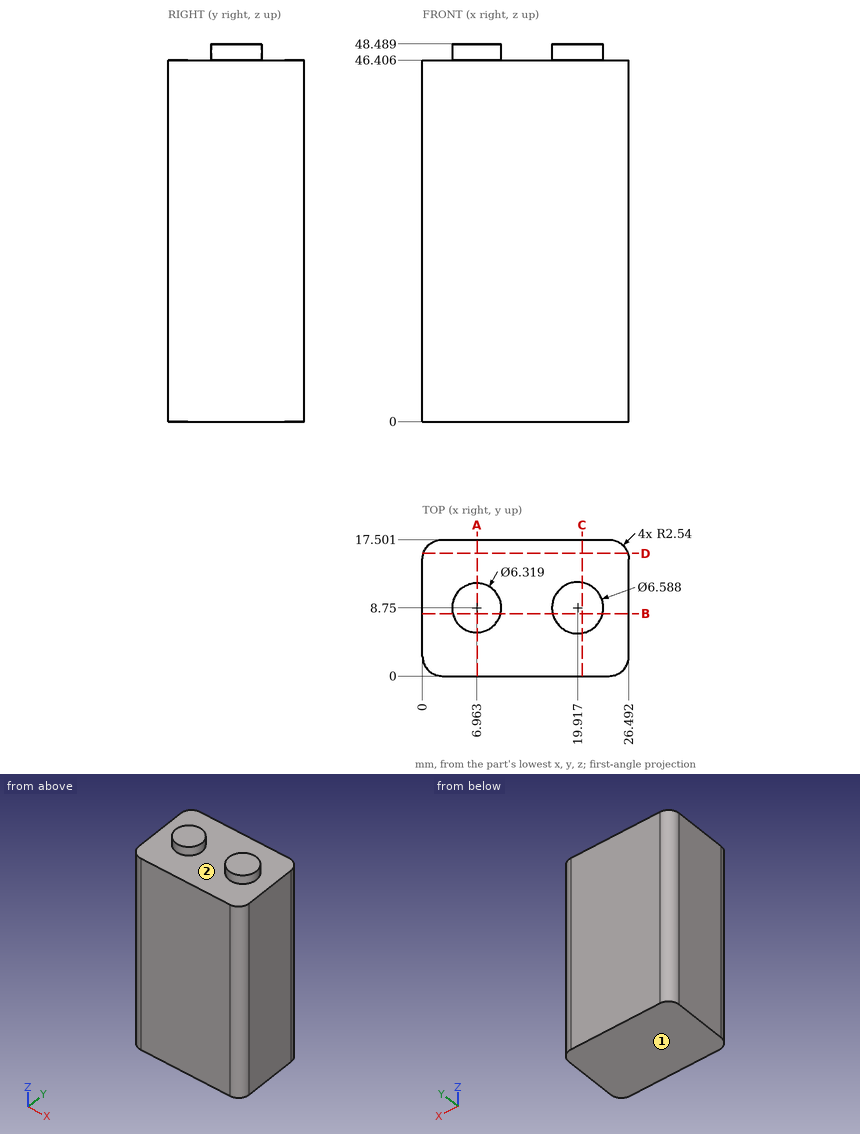
Verification items for this drawing (mm, ordinates from the low corner). A direction names the side the tool comes from. Round coordinates to 2 decimals unless told otherwise and drop trailing zeros. Order: outer loops, then holes, each group sorted by start corner. A loop starts at its lowest first (then second) coordinate and runs counter-clockwise, first axis right, second up. Notation, with made-up numbers: (20.25, 68) - (26.25, 68) arc R25 ccw to (26.25, 88) - close; hole circle Ø11 at (34.5, 8). An arc over 180 degrees is marked (long way). Use CSV: the item, a comma, the result in double quotes. Start each with the question number.
1) Section check D-D, the plane y = 15.75. Record the cut outline in (x, z) (1 decimal).
2) Section check C-C, the plane x = 20.5. Record the cut outline in (y, z) (1 decimal), plus the area to 3 significant figures.
3) Access from +Z, -Z, +X, -X, +Y, -Y to the whole of each face (thin tool, end or side, straight path). Record for the marked faces 1 and 2.
4) Thickness scan on L1, parallel to Z at x = 22.5, y = 2 (1 decimal); L2, parallel to X at y = 1, z = 24; L3, parallel to X at y = 0.5, z = 27 (1 decimal). Record the ranges inside material, lowest first.
5) Section check B-B, the plane y = 8. Record the cut outline in (x, z) (1 decimal), plus the area to 3 significant figures.
6) Section check A-A, the plane x = 7. Record the cut outline in (y, z) (1 decimal).
Answers:
1,outline,"(0.1, 0) - (26.4, 0) - (26.4, 46.4) - (0.1, 46.4) - close"
2,outline,"(0, 0) - (17.5, 0) - (17.5, 46.4) - (12, 46.4) - (12, 48.5) - (5.5, 48.5) - (5.5, 46.4) - (0, 46.4) - close"
2,area,"826 mm²"
3,face 1,"-Z, +X, -X, +Y, -Y"
3,face 2,"+Z"
4,L1,"z = 0 to 46.4"
4,L2,"x = 0.52 to 25.97"
4,L3,"x = 1 to 25.5"
5,outline,"(0, 0) - (26.5, 0) - (26.5, 46.4) - (23.1, 46.4) - (23.1, 48.5) - (16.7, 48.5) - (16.7, 46.4) - (10, 46.4) - (10, 48.5) - (3.9, 48.5) - (3.9, 46.4) - (0, 46.4) - close"
5,area,"1,260 mm²"
6,outline,"(0, 0) - (17.5, 0) - (17.5, 46.4) - (11.9, 46.4) - (11.9, 48.5) - (5.6, 48.5) - (5.6, 46.4) - (0, 46.4) - close"
